Autodesk Inventor part; units mm, degrees
ref_plane "Work Plane1" through (-9, -9, 1.25) normal (0, 0, 1) x (1, 0, 0)
ref_plane "YZ Plane" through (0, 0, 0) normal (1, 0, 0) x (0, 1, 0)
ref_plane "XZ Plane" through (0, 0, 0) normal (0, 1, 0) x (-1, 0, 0)
sketch "Sketch1" plane through (0, 0, 0) normal (0, 0, 1) x (1, 0, 0)
  arc A0 (0, 9) -> (-7.7942, 4.5) centre (0, 0) ccw
  arc A1 (-5.0533, 10.5526) -> (0, 9) centre (0, 18) ccw
  arc A2 (-5.0533, 10.5526) -> (-6.6121, 9.6526) centre (-5.6148, 9.7251) ccw
  arc A3 (-7.7942, 4.5) -> (-6.6121, 9.6526) centre (-15.5885, 9) ccw
  arc A4 (7.7942, 4.5) -> (0, 9) centre (0, 0) ccw
  arc A5 (6.6121, 9.6526) -> (7.7942, 4.5) centre (15.5885, 9) ccw
  arc A6 (6.6121, 9.6526) -> (5.0533, 10.5526) centre (5.6148, 9.7251) ccw
  arc A7 (0, 9) -> (5.0533, 10.5526) centre (0, 18) ccw
  arc A8 (7.7942, -4.5) -> (7.7942, 4.5) centre (0, 0) ccw
  arc A9 (11.6654, -0.9) -> (7.7942, -4.5) centre (15.5885, -9) ccw
  arc A10 (11.6654, -0.9) -> (11.6654, 0.9) centre (11.2296, 0) ccw
  arc A11 (7.7942, 4.5) -> (11.6654, 0.9) centre (15.5885, 9) ccw
  arc A12 (0, -9) -> (7.7942, -4.5) centre (0, 0) ccw
  arc A13 (5.0533, -10.5526) -> (0, -9) centre (0, -18) ccw
  arc A14 (5.0533, -10.5526) -> (6.6121, -9.6526) centre (5.6148, -9.7251) ccw
  arc A15 (7.7942, -4.5) -> (6.6121, -9.6526) centre (15.5885, -9) ccw
  arc A16 (-7.7942, -4.5) -> (0, -9) centre (0, 0) ccw
  arc A17 (-6.6121, -9.6526) -> (-7.7942, -4.5) centre (-15.5885, -9) ccw
  arc A18 (-6.6121, -9.6526) -> (-5.0533, -10.5526) centre (-5.6148, -9.7251) ccw
  arc A19 (0, -9) -> (-5.0533, -10.5526) centre (0, -18) ccw
  arc A20 (-7.7942, 4.5) -> (-7.7942, -4.5) centre (0, 0) ccw
  arc A21 (-11.6654, 0.9) -> (-7.7942, 4.5) centre (-15.5885, 9) ccw
  arc A22 (-11.6654, 0.9) -> (-11.6654, -0.9) centre (-11.2296, 0) ccw
  arc A23 (-7.7942, -4.5) -> (-11.6654, -0.9) centre (-15.5885, -9) ccw
  circle A24 centre (0, 0) radius 6.5
  point P0 (0, 0)
ref_plane "Work Plane1" through (-9, -9, 1.25) normal (0, 0, 1) x (1, 0, 0)
extrude "Extrusion1" add sketch "Sketch1" along normal up to surface (1.25 mm away)
properties part number "piece-fixer"
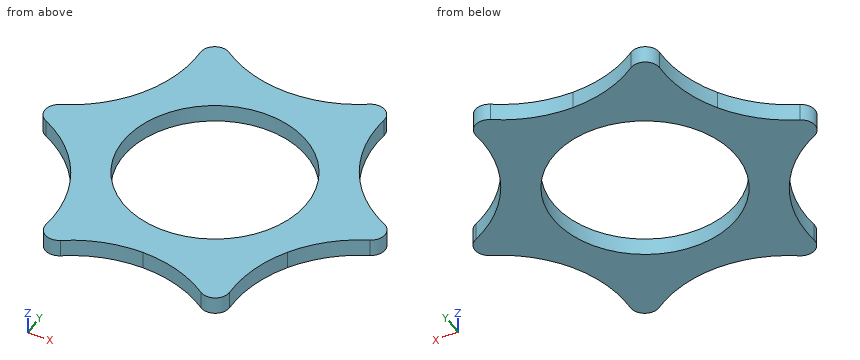
Could you check a few things on this model? Use its own coordinates, in mm. Coordinates: 2 decimals unless noted, no trailing zeros. Loops run counter-clockwise (first coordinate to the right, second up) from the corner with the lowest first, then second, coordinate; pieces in that order, holes last.
1) Imagine slicing it at C-C (z = 0.6). List the corners of the cut face in (x, y) for me, and give its area (3 significant figures).
Reported:
outline: (-11.67, -0.9) arc R9 cw to (-7.79, -4.5) arc R9 cw to (-6.61, -9.65) arc R1 ccw to (-5.05, -10.55) arc R9 cw to (0, -9) arc R9 cw to (5.05, -10.55) arc R1 ccw to (6.61, -9.65) arc R9 cw to (7.79, -4.5) arc R9 cw to (11.67, -0.9) arc R1 ccw to (11.67, 0.9) arc R9 cw to (7.79, 4.5) arc R9 cw to (6.61, 9.65) arc R1 ccw to (5.05, 10.55) arc R9 cw to (0, 9) arc R9 cw to (-5.05, 10.55) arc R1 ccw to (-6.61, 9.65) arc R9 cw to (-7.79, 4.5) arc R9 cw to (-11.67, 0.9) arc R1 ccw to start; hole circle Ø13 at (0, 0)
area: 191 mm2
2) Please list where these lines run through material, in increasing order: line 1 along Y through (x, z) = (0, 0.95); line 2 along Y through (x, z) = (-7.5, 1.1); line 3 along Y through (x, z) = (-1, 0.1).
Reported:
line 1: y = -9 to -6.5, 6.5 to 9
line 2: y = -5.05 to 5.05
line 3: y = -9.06 to -6.42, 6.42 to 9.06
3) Imagine slicing it at A-A (x = 4). List the corners of the cut face in (y, z) for me.
Reported:
outline: (-9.94, 0) - (-5.12, 0) - (-5.12, 1.25) - (-9.94, 1.25) - close; (5.12, 0) - (9.94, 0) - (9.94, 1.25) - (5.12, 1.25) - close
4) Imagine slicing it at D-D (y = 7.5). List the corners of the cut face in (x, z) for me.
Reported:
outline: (-6.71, 0) - (6.71, 0) - (6.71, 1.25) - (-6.71, 1.25) - close
5) Imagine slicing it at B-B (y = 2.5). List the corners of the cut face in (x, z) for me.
Reported:
outline: (-9.36, 0) - (-6, 0) - (-6, 1.25) - (-9.36, 1.25) - close; (6, 0) - (9.36, 0) - (9.36, 1.25) - (6, 1.25) - close
